```python
from build123d import *

# Parameters (mm, degrees)
SKETCH1_R           = 7.5
BOSS_EXTRUDE1_DEPTH = 47.5
SKETCH2_R           = 8
BOSS_EXTRUDE2_DEPTH = 2
SKETCH3_W           = 1.1
SKETCH3_H           = 0.35
CHAMFER1_SIZE       = 0.4


with BuildPart() as part:
    # Sketch1 → Boss-Extrude1 (new, symmetric)
    with BuildSketch(Plane(origin=(0, 0, 0), x_dir=(0, 0, -1), z_dir=(1, 0, 0))):
        Circle(SKETCH1_R)
    extrude(amount=BOSS_EXTRUDE1_DEPTH, both=True)

    # Sketch2 → Boss-Extrude2 (add)
    with BuildSketch(Plane(origin=(47.5, 0, 0), x_dir=(0, 0, -1), z_dir=(1, 0, 0))):
        Circle(SKETCH2_R)
    extrude(amount=BOSS_EXTRUDE2_DEPTH)

    # Sketch3 → Cut-Revolve1 (revolve, cut)
    with BuildSketch(Plane(origin=(0, 0, 0), x_dir=(1, 0, 0), z_dir=(0, 1, 0))):
        with Locations((-43.65, 7.325)):
            Rectangle(SKETCH3_W, SKETCH3_H)
    revolve(axis=Axis((0, 0, 0), (-1, 0, 0)), mode=Mode.SUBTRACT)

    # Chamfer1
    chamfer1_edges = [part.edges().sort_by_distance(p)[0] for p in [
        (-47.5, 0, 7.5),
        (49.5, 0, 8),
    ]]
    chamfer(chamfer1_edges, length=CHAMFER1_SIZE)


solid = part.part
```
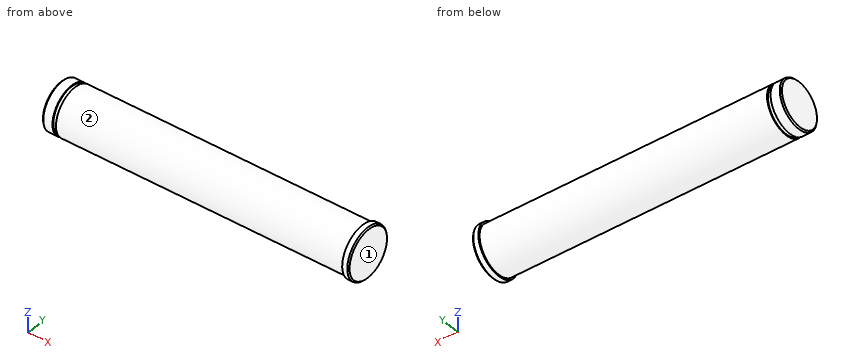
Geometry check sheet. Reference: the model listing, model coordinates, mm. Face numbers are marked on the shaded views. A direction names the side the tool comes from. Coordinates: 2 decimals unless noted, no trailing zeros. Order: outer loops, then holes, each group sorted by start corner. A loop starts at its lowest first (then second) coordinate and runs counter-clockwise, first axis right, second up.
Q1. Sectioned sample at A-A on y = 0. Record the cut outline in (x, z), and give its area (3 significant figures).
Reply:
outline: (-47.5, -7.1) - (-47.1, -7.5) - (-44.2, -7.5) - (-44.2, -7.15) - (-43.1, -7.15) - (-43.1, -7.5) - (47.5, -7.5) - (47.5, -8) - (49.1, -8) - (49.5, -7.6) - (49.5, 7.6) - (49.1, 8) - (47.5, 8) - (47.5, 7.5) - (-43.1, 7.5) - (-43.1, 7.15) - (-44.2, 7.15) - (-44.2, 7.5) - (-47.1, 7.5) - (-47.5, 7.1) - close
area: 1,460 mm2
Q2. Thickness scan on probe 1 along X at (y, z) = (-7, -2.5); probe 2 along X at (y, z) = (-6.75, 2.5); probe 3 along Y at (x, z) = (7.5, 4.25). Record the ranges inside material, lowest first.
Reply:
probe 1: x = -47.17 to -44.2, -43.1 to 49.5
probe 2: x = -47.4 to -44.2, -43.1 to 49.5
probe 3: y = -6.18 to 6.18
Q3. Depth check by flat-ended pin: pin 1 Ø6 at (x, z) = (38, -1.5) entering from -Y; pin 2 Ø1.5 at (x, y) = (-13.5, 2.5) entering from -Z; pin 3 Ø3 at (x, z) = (18, -4.5) entering from -Y. Enter the tip coordinate at first touch or a pass-through.
Reply:
pin 1: stops at y = -7.5
pin 2: stops at z = -7.29
pin 3: stops at y = -6.87
Q4. Tool access check on the marked faces 1 and 2. Record the directions out of +Z, -Z, +X, -X, +Y, -Y that give a thin tool (end or side, any length) a straight path to the whole face; none if there is none.
Reply:
face 1: +Z, -Z, +X, +Y, -Y
face 2: -X
Q5. Sectioned sample at C-C on x = -36. Record the cut outline in (y, z), and give its area (3 significant figures).
Reply:
outline: circle Ø15 at (0, 0)
area: 177 mm2
